Build history of the part. All positions in model axes, mm. A direction names the side the tool comes from. Give positions to 0.01 mm unless a question says otherwise; leave off trailing zeros. Order: outer loops, then holes, each group sorted by start corner. A loop starts at its lowest first (then second) coordinate and runs counter-clockwise, first axis right, second up. Notation, with made-up numbers: M 4,55 L 12,55 A28 ccw 12,94 Z; hole C -22.75,-32.5 d2. An arc over 180 degrees is marked long. Answer as CSV lines item,"result".
from build123d import *

# Parameters (mm, degrees)
SKIZZE1_W                       = 43
SKIZZE1_H                       = 95
AUFSATZ_LINEAR_AUSTRAGEN1_DEPTH = 20
SKIZZE2_R                       = 13
SCHNITT_LINEAR_AUSTRAGEN1_DEPTH = 34
SKIZZE3_R                       = 9.5
SCHNITT_LINEAR_AUSTRAGEN2_DEPTH = 34
SKIZZE4_W                       = 20
SKIZZE4_H                       = 3
SCHNITT_LINEAR_AUSTRAGEN3_DEPTH = 15
SKIZZE8_R                       = 1.62
SCHNITT_LINEAR_AUSTRAGEN6_DEPTH = 5
SKIZZE9_R                       = 1.62
SCHNITT_LINEAR_AUSTRAGEN7_DEPTH = 5
SKIZZE10_R                      = 1.5
SCHNITT_LINEAR_AUSTRAGEN8_DEPTH = 12
SKIZZE11_W                      = 20
SKIZZE11_H                      = 95
AUFSATZ_LINEAR_AUSTRAGEN2_DEPTH = 2


with BuildPart() as part:
    # Skizze1 → Aufsatz-Linear austragen1 (new body)
    with BuildSketch(Plane.XY):
        with Locations((21.5, 47.5)):
            Rectangle(SKIZZE1_W, SKIZZE1_H)
    extrude(amount=AUFSATZ_LINEAR_AUSTRAGEN1_DEPTH)

    # Skizze2 → Schnitt-Linear austragen1 (cut)
    with BuildSketch(Plane.XY.offset(20)):
        with Locations((21.85, 15)):
            Circle(SKIZZE2_R)
    extrude(amount=-SCHNITT_LINEAR_AUSTRAGEN1_DEPTH, mode=Mode.SUBTRACT)

    # Skizze3 → Schnitt-Linear austragen2 (cut)
    with BuildSketch(Plane.XY.offset(20)):
        with Locations((21.85, 65)):
            Circle(SKIZZE3_R)
    extrude(amount=-SCHNITT_LINEAR_AUSTRAGEN2_DEPTH, mode=Mode.SUBTRACT)

    # Skizze4 → Schnitt-Linear austragen3 (cut)
    with BuildSketch(Plane(origin=(0, 95, 0), x_dir=(1, 0, 0), z_dir=(0, 1, 0))):
        with Locations((33, -1.5)):
            Rectangle(SKIZZE4_W, SKIZZE4_H)
    extrude(amount=-SCHNITT_LINEAR_AUSTRAGEN3_DEPTH, mode=Mode.SUBTRACT)

    # Skizze8 → Schnitt-Linear austragen6 (cut)
    with BuildSketch(Plane(origin=(0, 0, 3), x_dir=(-1, 0, 0), z_dir=(0, 0, -1))):
        with Locations((-38, 86)):
            Circle(SKIZZE8_R)
    extrude(amount=-SCHNITT_LINEAR_AUSTRAGEN6_DEPTH, mode=Mode.SUBTRACT)

    # Skizze9 → Schnitt-Linear austragen7 (cut)
    with BuildSketch(Plane(origin=(0, 0, 3), x_dir=(-1, 0, 0), z_dir=(0, 0, -1))):
        with Locations((-28, 86)):
            Circle(SKIZZE9_R)
    extrude(amount=-SCHNITT_LINEAR_AUSTRAGEN7_DEPTH, mode=Mode.SUBTRACT)

    # Skizze10 → Schnitt-Linear austragen8 (cut)
    with BuildSketch(Plane(origin=(0, 0, 0), x_dir=(-1, 0, 0), z_dir=(0, 0, -1))):
        with Locations((-4.35, 15)):
            Circle(SKIZZE10_R)
        with Locations((-39.35, 15)):
            Circle(SKIZZE10_R)
    extrude(amount=-SCHNITT_LINEAR_AUSTRAGEN8_DEPTH, mode=Mode.SUBTRACT)

    # Skizze11 → Aufsatz-Linear austragen2 (add)
    with BuildSketch(Plane.ZY):
        with Locations((10, 47.5)):
            Rectangle(SKIZZE11_W, SKIZZE11_H)
    extrude(amount=AUFSATZ_LINEAR_AUSTRAGEN2_DEPTH)


solid = part.part
Item 1: Pull direction Y, two halves, no side cores. Call faces 4 (the flat face through (33, 80, 1)), 5 (the flat face through (28, 86, 8)), 6 (the flat face through (21, 0, 10)): released by +Y, released by -Y, zero draft, split by the parting line, or undercut.
Geometry says:
face 4,"released by +Y"
face 5,"undercut"
face 6,"released by -Y"
Item 2: Probe line 1 along Y through (x, z) = (21.85, 4); line 2 along X through (y, z) = (86, 5.3); line 3 along Y through (x, z) = (16.5, 7). List the from-to ranges inside material, lowest first. Write a range as from..to.
Geometry says:
line 1,"y = 0..2, 28..55.5, 74.5..95"
line 2,"x = -2..26.38, 29.62..36.38, 39.62..43"
line 3,"y = 0..3.15, 26.85..57.15, 72.85..95"
Item 3: Band-saw the part on C-C (z = 5.5). Give the cut face in (x, y), and give its area (3 significant figures).
Geometry says:
outline,"M -2,0 L 43,0 L 43,95 L -2,95 Z; hole C 4.35,15 d3; hole C 21.85,15 d26; hole C 21.85,65 d19; hole C 28,86 d3.24; hole C 38,86 d3.24; hole C 39.35,15 d3"
area,"3,430 mm2"
Item 4: Band-saw the part on D-D (y = 86). Give the cut face in (x, z), and give its area (3 significant figures).
Geometry says:
outline,"M -2,0 L 23,0 L 23,3 L 26.38,3 L 26.38,8 L 29.62,8 L 29.62,3 L 36.38,3 L 36.38,8 L 39.62,8 L 39.62,3 L 43,3 L 43,20 L -2,20 Z"
area,"808 mm2"
Item 5: Band-saw the part on B-B (x = 21.85). Give the cut face in (y, z).
Geometry says:
outline,"M 0,0 L 2,0 L 2,20 L 0,20 Z; M 28,0 L 55.5,0 L 55.5,20 L 28,20 Z; M 74.5,0 L 95,0 L 95,20 L 74.5,20 Z"
Item 6: 3-axis set-ups, long thin cutter, end or side, ignore diameter. For faces 1 (the flat face through (-2, 48, 10)), 2 (the flat face through (33, 88, 3)), 3 (the cylindrical face through (29.194, 87.095, 5.465)): which of +Z, -Z, +X, -X, +Y, -Y reach the whole face in a straight line?
Geometry says:
face 1,"+Z, -Z, -X, +Y, -Y"
face 2,"-Z, +X, +Y"
face 3,"-Z"
Item 7: Band-saw the part on A-A (y = 15). Give the cut face in (x, z), and give its area (3 significant figures).
Geometry says:
outline,"M -2,0 L 2.85,0 L 2.85,12 L 5.85,12 L 5.85,0 L 8.85,0 L 8.85,20 L -2,20 Z; M 34.85,0 L 37.85,0 L 37.85,12 L 40.85,12 L 40.85,0 L 43,0 L 43,20 L 34.85,20 Z"
area,"308 mm2"
Item 8: Drop flat-ended pins along their axis: pin 1 (16.5 mm diameter, centred on x = 32, y = 89, fed in from -Z); pin 2 (1.5 mm diameter, centred on x = 34, z = 2, fed in from +Y); pin 3 (3.5 mm diameter, centred on y = 84, z = 1, fed in from +X); pin 4 (17 mm diameter, centred on x = 21.85, y = 65, fed in from +Z). Give the stop position or say it passes through.
Geometry says:
pin 1,"stops at z = 3"
pin 2,"stops at y = 80"
pin 3,"stops at x = 23"
pin 4,"passes through"
